Autodesk Inventor part; units mm, degrees
ref_plane "YZ Plane" through (0, 0, 0) normal (1, 0, 0) x (0, 1, 0)
ref_plane "XZ Plane" through (0, 0, 0) normal (0, 1, 0) x (-1, 0, 0)
ref_plane "XY Plane" through (0, 0, 0) normal (0, 0, 1) x (1, 0, 0)
sketch "Sketch4" plane through (0, 0, 0) normal (1, 0, 0) x (0, 1, 0)
  line L0 (6, 7.6) -> (3, 7.6)
  line L1 (3, 7.6) -> (3, 5.6)
  line L2 (3, 5.6) -> (0, 5.6)
  line L3 (0, 0) -> (3, 0)
  line L4 (3, 0) -> (3, -2)
  line L5 (3, -2) -> (6, -2)
  line L6 (6, -2) -> (6, 7.6)
  line L7 (8, 10.6) -> (0, 10.6)
  line L8 (0, 10.6) -> (0, 7.8)
  line L9 (0, 7.8) -> (0, 7.8)
  line L10 (0, -4.2) -> (8, -4.2)
  line L11 (8, -4.2) -> (8, 10.6)
  line L12 (0, 7.8) -> (0, 5.6)
  line L13 (0.2401, 0) -> (0, 0)
  line L14 (0, 0) -> (0, -4.2)
  point P0 (4.5, 7.6)
  dimension "d23" = 2
  dimension "d24" = 3
  dimension "d28" = 2
  dimension "d29" = 5.6
  dimension "d31" = 3
extrude "Extrusion3" add sketch "Sketch4" along normal blind 10
fillet "Fillet6" radius 1.5 2 edges at (5, 0, 5.6) (5, 0, 0)
properties part number "guia"
Geometry check sheet. Reference: the model listing, model coordinates, mm. A direction names the side the tool comes from. Round coordinates to 2 decimals unless told otherwise and drop trailing zeros. Order: outer loops, then holes, each group sorted by start corner. A loop starts at its lowest first (then second) coordinate and runs counter-clockwise, first axis right, second up. Notation, with made-up numbers: (76, -29) -> (100, -29) arc R21 ccw to (100, 7) -> close; hole circle Ø5 at (2, 0.5). An arc over 180 degrees is marked (long way). Use one line per item in the form item = value.
1. Cross-section at B-B, the plane z = -1.75. Enter the section's corners in (x, y), plus the area to 3 significant figures.
Working result:
outline = (0, 0) -> (10, 0) -> (10, 3) -> (0, 3) -> close; (0, 6) -> (10, 6) -> (10, 8) -> (0, 8) -> close
area = 50.0 mm^2
2. Cross-section at A-A, the plane y = 3.25. Enter the section's corners in (x, z).
Working result:
outline = (0, -4.2) -> (10, -4.2) -> (10, -2) -> (0, -2) -> close; (0, 7.6) -> (10, 7.6) -> (10, 10.6) -> (0, 10.6) -> close
3. Cross-section at C-C, the plane z = 4. Enter the section's corners in (x, y).
Working result:
outline = (0, 6) -> (10, 6) -> (10, 8) -> (0, 8) -> close
4. Scan lines: line 1 along Z through (x, y) = (9.5, 2.25); line 2 along Z through (x, y) = (3.5, 4.25); line 3 along Y through (x, z) = (6, 5). Record each from-to range of solid material in increasing order. Write a range as from..to.
Working result:
line_1 = -4.2..0, 5.6..10.6
line_2 = -4.2..-2, 7.6..10.6
line_3 = 6..8
5. Go/stop test with flat-tipped pins: pin 1 (2 mm diameter, centred on x = 7, z = 4, fed in from -Y); pin 2 (2 mm diameter, centred on y = 2, z = -2.5, fed in from -X); pin 3 (3 mm diameter, centred on x = 6, z = 4.5, fed in from -Y). Record where each tip stops, or that it passes through.
Working result:
pin_1 = 6
pin_2 = 0
pin_3 = 0.48
6. Set-up check for faces 4 (the face through (5, 2, 0)), 5 (the face through (5, 4, -2)), 6 (the face through (10, 7, 3)): record each of +Z, -Z, +X, -X, +Y, -Y from which the full face is reachable in a straight line by a thin tool's end or side.
Working result:
face_4 = +X, -X, -Y
face_5 = +X, -X
face_6 = +Z, -Z, +X, +Y, -Y
7. Mould release check, pull along Y, two halves, no side actions. Record for faces 1 (the face through (5, 2, 5.6)), 2 (the face through (5, 6, 3)), 3 (the face through (5, 8, 3)): pulls with the +Y half, pulls with the -Y half, needs draft (parallel to the pull), parting line crosses it, or undercut.
Working result:
face_1 = needs draft
face_2 = undercut
face_3 = pulls with the +Y half
